Input: part model. Units: mm. Frame: model coordinates. Face numbers are marked on the shaded views. A direction names the side the tool comes from. Give positions to 0.01 mm unless a question says otherwise; leave off trailing zeros. Order: outer loops, then holes, each group sorted by start corner. A loop starts at its lowest first (then second) coordinate and runs counter-clockwise, first axis right, second up. Notation, with made-up numbers: M 51,72.25 L 57,72.25 A13 cw 57,77.25 Z; hole C -40,-19.75 d9. An arc over 180 degrees is marked long. Use a Markdown table: item, result.
from build123d import *

# Parameters (mm, degrees)
F1_DEPTH = 25.4
F2_W     = 203.2
F2_H     = 50.8
F3_DEPTH = 76.2
F4_W     = 101.6
F4_H     = 50.8
F5_DEPTH = 25.4
F7_DEPTH = 50.8
F9_DEPTH = 50.8


with BuildPart() as f1:
    # F0 (on Top) → F1 (new body)
    with BuildSketch(Plane.XY):
        Polygon((101.6, -50.8), (101.6, 50.8), (-101.6, 50.8), (-101.6, -50.8), (-50.8, -50.8), (-50.8, -25.4), (50.8, -25.4), (50.8, -50.8), align=None)
    extrude(amount=F1_DEPTH)

    # F2 (on face) → F3 (join)
    with BuildSketch(Plane.XY.offset(25.4)):
        with Locations((0, 25.4)):
            Rectangle(F2_W, F2_H)
    extrude(amount=F3_DEPTH)

    # F4 (on face) → F5 (cut)
    with BuildSketch(Plane.XY.offset(101.6)):
        with Locations((0, 25.4)):
            Rectangle(F4_W, F4_H)
    extrude(amount=-F5_DEPTH, mode=Mode.SUBTRACT)

    # F6 (on face) → F7 (cut)
    with BuildSketch(Plane.XZ):
        Polygon((101.6, 101.6), (76.2, 101.6), (101.6, 76.2), align=None)
    extrude(amount=-F7_DEPTH, mode=Mode.SUBTRACT)

    # F8 (on face) → F9 (cut)
    with BuildSketch(Plane.XZ):
        Polygon((-101.6, 76.2), (-76.2, 101.6), (-101.6, 101.6), align=None)
    extrude(amount=-F9_DEPTH, mode=Mode.SUBTRACT)


solid = f1.part
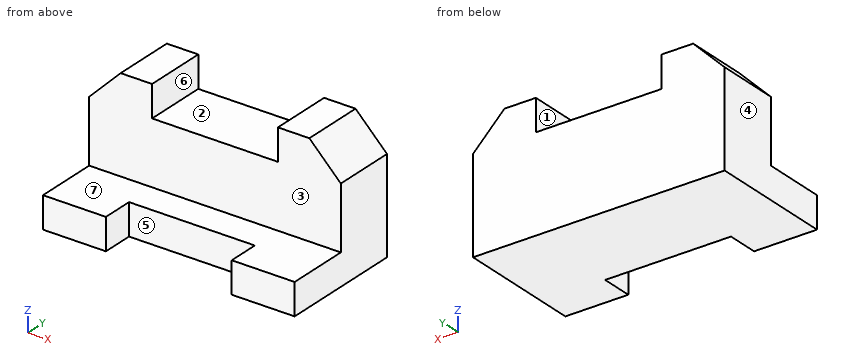
1) Mould query, pull axis X, two halves, no side actions, for the marked faces 1, 2, 3 and 4. Classes: released by +X, released by -X, zero draft, split by the parting line, or undercut.
Response values:
| item | result |
|---|---|
| face 1 | undercut |
| face 2 | undercut |
| face 3 | zero draft |
| face 4 | released by -X |
2) Cut plane A-A on y = -36. Return loops of the section in (x, z), and give its area (3 significant figures).
Response values:
| item | result |
|---|---|
| outline | M -101.6,0 L -50.8,0 L -50.8,25.4 L -101.6,25.4 Z; M 50.8,0 L 101.6,0 L 101.6,25.4 L 50.8,25.4 Z |
| area | 2,580 mm² |
3) Reachability of the marked faces 5, 6 and 7 from +Z, -Z, +X, -X, +Y, -Y: full face, straight path, thin tool, end or side. Return the list, or none.
Response values:
| item | result |
|---|---|
| face 5 | +Z, -Z, -Y |
| face 6 | +Z, +Y, -Y |
| face 7 | +Z, +X, -X, -Y |
4) Cut plane B-B on y = 12.5. Return loops of the section in (x, z).
Response values:
| item | result |
|---|---|
| outline | M -101.6,0 L 101.6,0 L 101.6,76.2 L 76.2,101.6 L 50.8,101.6 L 50.8,76.2 L -50.8,76.2 L -50.8,101.6 L -76.2,101.6 L -101.6,76.2 Z |
5) First-contact query: pin 1 Ø15 at (x, y) = (22.5, 33) entering from +Z; pin 2 Ø12.5 at (y, z) = (22.5, 90) entering from -X; pin 3 Ø20.5 at (x, z) = (15, 16.5) entering from -Y; pin 4 Ø10 at (x, z) = (26, 82.5) entering from -Y. Flat tips, straight axial feed; report the tip coordinate or a pass-through.
Response values:
| item | result |
|---|---|
| pin 1 | stops at z = 76.2 |
| pin 2 | stops at x = -94.05 |
| pin 3 | stops at y = -25.4 |
| pin 4 | passes through |
6) Material intervals for line 1 (X direction, y = -42.5, z = 22); line 2 (Y direction, x = 46, z = 19); line 3 (Y direction, x = 3.5, z = 43), sorted ascending. Write a range as from..to.
Response values:
| item | result |
|---|---|
| line 1 | x = -101.6..-50.8, 50.8..101.6 |
| line 2 | y = -25.4..50.8 |
| line 3 | y = 0..50.8 |
7) Cut plane D-D on z = 12. Return loops of the section in (x, y), and give its area (3 significant figures).
Response values:
| item | result |
|---|---|
| outline | M -101.6,-50.8 L -50.8,-50.8 L -50.8,-25.4 L 50.8,-25.4 L 50.8,-50.8 L 101.6,-50.8 L 101.6,50.8 L -101.6,50.8 Z |
| area | 18,100 mm² |
8) Cut plane C-C on x = -66.5. Return loops of the section in (y, z), and give its area (3 significant figures).
Response values:
| item | result |
|---|---|
| outline | M -50.8,0 L 50.8,0 L 50.8,101.6 L 0,101.6 L 0,25.4 L -50.8,25.4 Z |
| area | 6,450 mm² |
